Design review of the part built by this model. Coordinates are the model's own, in mm. A direction names the side the tool comes from. Give positions to 0.01 mm unless a question says otherwise; leave off trailing zeros. Order: outer loops, then holes, each group sorted by start corner. A loop starts at its lowest first (then second) coordinate and runs counter-clockwise, first axis right, second up. Notation, with made-up numbers: M 55.25,-25.5 L 86.25,-25.5 A5 cw 86.25,-19.5 Z; hole C 16,-3 d2. An arc over 180 degrees is marked long. Answer as a JSON object with one key per item and string values.
from build123d import *

# Parameters (mm, degrees)
SKETCH_1_W          = 150
SKETCH_1_H          = 100
SKETCH_1_R          = 1.6
EXTRUDE_1_DEPTH     = 3
SKETCH_2_W          = 45.012904103
SKETCH_2_H          = 5.754361308
SKETCH_2_W_2        = 7.270480745
SKETCH_2_W_3        = 7.901217153
SKETCH_2_H_2        = 17.152026815
EXTRUDE_2_DEPTH     = 30
CUT_EXTRUDE_1_DEPTH = 5


with BuildPart() as part:
    # 草图1 → 凸台-拉伸1 (new body)
    with BuildSketch(Plane.XY):
        with Locations((18.212237094, -8.671684116)):
            Rectangle(SKETCH_1_W, SKETCH_1_H)
        with Locations((-46.787762906, 31.328315884)):
            Circle(SKETCH_1_R, mode=Mode.SUBTRACT)
        with Locations((-46.787762906, 11.328315884)):
            Circle(SKETCH_1_R, mode=Mode.SUBTRACT)
        with Locations((83.212237094, 11.328315884)):
            Circle(SKETCH_1_R, mode=Mode.SUBTRACT)
        with Locations((83.212237094, 31.328315884)):
            Circle(SKETCH_1_R, mode=Mode.SUBTRACT)
    extrude(amount=EXTRUDE_1_DEPTH)

    # 草图2 → 凸台-拉伸2 (add)
    with BuildSketch(Plane.XY.offset(3)):
        with Locations((18.854591116, 38.45113523)):
            Rectangle(SKETCH_2_W, SKETCH_2_H)
        with Locations((-53.152522534, 38.45113523)):
            Rectangle(SKETCH_2_W_2, SKETCH_2_H)
        with Locations((89.261628518, 38.45113523)):
            Rectangle(SKETCH_2_W_3, SKETCH_2_H)
        with Locations((89.261628518, -50.095670709)):
            Rectangle(SKETCH_2_W_3, SKETCH_2_H_2)
        with Locations((-53.152522534, -50.095670709)):
            Rectangle(SKETCH_2_W_2, SKETCH_2_H_2)
    extrude(amount=EXTRUDE_2_DEPTH)

    # 草图3 → 切除-拉伸1 (cut)
    with BuildSketch(Plane(origin=(0, 0, 0), x_dir=(-1, 0, 0), z_dir=(0, 0, -1))):
        with BuildLine():
            Line((-58.212237094, -37.071684116), (21.787762906, -37.071684116))
            ThreePointArc((21.787762906, -37.071684116), (23.387762906, -38.671684116), (21.787762906, -40.271684116))
            Line((21.787762906, -40.271684116), (-58.212237094, -40.271684116))
            ThreePointArc((-58.212237094, -40.271684116), (-59.812237094, -38.671684116), (-58.212237094, -37.071684116))
        make_face()
        with BuildLine():
            Line((-58.212237094, -47.071684116), (21.787762906, -47.071684116))
            ThreePointArc((21.787762906, -47.071684116), (23.387762906, -48.671684116), (21.787762906, -50.271684116))
            Line((21.787762906, -50.271684116), (-58.212237094, -50.271684116))
            ThreePointArc((-58.212237094, -50.271684116), (-59.812237094, -48.671684116), (-58.212237094, -47.071684116))
        make_face()
    extrude(amount=-CUT_EXTRUDE_1_DEPTH, mode=Mode.SUBTRACT)


solid = part.part
(1) Draft analysis for pull direction Y (two halves, no side actions). For faces 1 (the cylindrical face through (82.033, 32.41, 1.479)), 2 (the flat face through (85.311, 38, 18)), 3 (the flat face through (18, -58.672, 2)), state which applies: +Y half, -Y half, draft (parallel to the pull), parting line (faces both ways), or undercut.
Checked values:
{"face 1": "undercut", "face 2": "draft", "face 3": "-Y half"}
(2) Insertion check: pin 1 (5 mm diameter, centred on x = -46.79, y = 31.33, fed in from +Z); pin 2 (12 mm diameter, centred on x = 27.5, z = 11, fed in from -Y). Each pin has a flat end and moves straight along its axis. Give the tip position at first contact, or say it passes through.
Checked values:
{"pin 1": "stops at z = 3", "pin 2": "stops at y = 35.57"}
(3) To check wall thickness, follow L1, parallel to Z at x = 62.5, y = -46.5; L2, parallel to Y at x = 13, z = 14. State the ranges of each line that lie inside material, in increasing order. Write a range as from..to.
Checked values:
{"L1": "z = 0..3", "L2": "y = 35.57..41.33"}
(4) Tool access review of faces 4 (the flat face through (41.361, 38, 18)), 5 (the cylindrical face through (59.81, -48.71, 1.48)), 6 (the flat face through (19, 35.574, 18)), 7 (the flat face through (-56.788, -27, 2)): name each direction out of +Z, -Z, +X, -X, +Y, -Y from which nothing blocks a thin tool from reaching the whole face with its end or side.
Checked values:
{"face 4": "+Z, +Y, -Y", "face 5": "+Z, -Z", "face 6": "+Z, +X, -X, -Y", "face 7": "+Z, -Z, -X, +Y, -Y"}
(5) We need section B-B (z = 23). Write out the cut boundary in (x, y).
Checked values:
{"outline": "M -56.79,-58.67 L -49.52,-58.67 L -49.52,-41.52 L -56.79,-41.52 Z; M -56.79,35.57 L -49.52,35.57 L -49.52,41.33 L -56.79,41.33 Z; M -3.65,35.57 L 41.36,35.57 L 41.36,41.33 L -3.65,41.33 Z; M 85.31,-58.67 L 93.21,-58.67 L 93.21,-41.52 L 85.31,-41.52 Z; M 85.31,35.57 L 93.21,35.57 L 93.21,41.33 L 85.31,41.33 Z"}
(6) We need section C-C (x = -18.5). Write out the cut boundary in (y, z).
Checked values:
{"outline": "M -58.67,0 L -50.27,0 L -50.27,3 L -58.67,3 Z; M -47.07,0 L -40.27,0 L -40.27,3 L -47.07,3 Z; M -37.07,0 L 41.33,0 L 41.33,3 L -37.07,3 Z"}
(7) We need section D-D (y = -17.5). Write out the cut boundary in (x, z), plus the area to 3 significant figures.
Checked values:
{"outline": "M -56.79,0 L 93.21,0 L 93.21,3 L -56.79,3 Z", "area": "450 mm^2"}
(8) We need section A-A (x = 20). Write out the cut boundary in (y, z).
Checked values:
{"outline": "M -58.67,0 L -50.27,0 L -50.27,3 L -58.67,3 Z; M -47.07,0 L -40.27,0 L -40.27,3 L -47.07,3 Z; M -37.07,0 L 41.33,0 L 41.33,33 L 35.57,33 L 35.57,3 L -37.07,3 Z"}
